Can you work these out from the model? Positions are in its coordinate system, mm. Coordinates: 2 decimals unless noted, no trailing zeros. Order: outer loops, then holes, each group sorted by start corner. A loop starts at its lowest first (then second) coordinate and runs counter-clockwise, first axis right, second up. Notation, with made-up numbers: (82.25, 34) -> (108.25, 34) arc R14 cw to (108.25, 55) -> close; hole circle Ø10 at (12, 6). An arc over 180 degrees is marked (long way). Return JSON: item names as keys, results as strings. Group by question number.
1) For pin 1 (1.6 mm diameter, centred on x = -10.5, z = 29.5, fed in from +Y); pin 2 (0.8 mm diameter, centred on y = -20.5, z = 29, fed in from -X); pin 3 (1.1 mm diameter, centred on y = -20.5, z = 29, fed in from +X); pin 4 (0.8 mm diameter, centred on x = 10.5, z = 29.5, fed in from +Y), each with a flat end and sliding along its axis, tell me the tip position at first contact or that it passes through.
2) If we section it at B-B, the plane y = 11: Please give me the cut outline in (x, z), then the cut area to 3 significant figures.
3) If we section it at A-A, the plane z = 29: Please give me the cut outline in (x, y), then the cut area to 3 significant figures.
4) If I drill on probe 1 along Y at (x, z) = (-12, 29.5), over which ranges is the centre line in solid material (lowest first)? Write a range as from..to.
from build123d import *

# Parameters (mm, degrees)
SKETCH_W        = 42
SKETCH_H        = 42
PAD_DEPTH       = 30
SKETCH001_W     = 40
SKETCH001_H     = 40
POCKET_DEPTH    = 1.5
SKETCH002_W     = 38
SKETCH002_H     = 38
POCKET001_DEPTH = 28
SKETCH003_W     = 10
SKETCH003_H     = 5
POCKET002_DEPTH = 300
SKETCH004_W     = 42
SKETCH004_H     = 42
PAD001_DEPTH    = 1.5


with BuildPart() as pocket002:
    # Sketch → Pad (new body)
    with BuildSketch(Plane.XY):
        Rectangle(SKETCH_W, SKETCH_H)
    extrude(amount=PAD_DEPTH)

    # Sketch001 → Pocket (cut)
    with BuildSketch(Plane.XY.offset(30)):
        Rectangle(SKETCH001_W, SKETCH001_H)
    extrude(amount=-POCKET_DEPTH, mode=Mode.SUBTRACT)

    # Sketch002 → Pocket001 (cut)
    with BuildSketch(Plane.XY.offset(28.5)):
        Rectangle(SKETCH002_W, SKETCH002_H)
    extrude(amount=-POCKET001_DEPTH, mode=Mode.SUBTRACT)

    # Sketch003 → Pocket002 (cut)
    with BuildSketch(Plane.XZ.offset(21)):
        with Locations((0, 27.5)):
            Rectangle(SKETCH003_W, SKETCH003_H)
    extrude(amount=-POCKET002_DEPTH, mode=Mode.SUBTRACT)


with BuildPart() as cut:
    # Pad001 base: copy of Pocket002
    add(pocket002.part)

    # Sketch004 → Pad001 (new body, symmetric)
    with BuildSketch(Plane.XY.offset(30)):
        Rectangle(SKETCH004_W, SKETCH004_H)
    extrude(amount=PAD001_DEPTH, both=True)

    # Cut: cut Pocket002
    add(pocket002.part, mode=Mode.SUBTRACT)


solid = cut.part
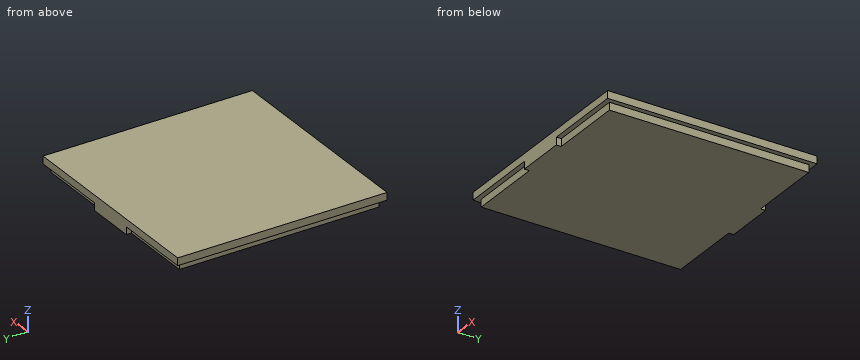
Result sheet:
{
 "1": {"pin 1": "stops at y = 21", "pin 2": "stops at x = -5", "pin 3": "stops at x = 20", "pin 4": "stops at y = 20"},
 "2": {"outline": "(-21, 30) -> (-20, 30) -> (-20, 28.5) -> (20, 28.5) -> (20, 30) -> (21, 30) -> (21, 31.5) -> (-21, 31.5) -> close", "area": "123 mm2"},
 "3": {"outline": "(-20, -20) -> (-5, -20) -> (-5, -21) -> (5, -21) -> (5, -20) -> (20, -20) -> (20, 20) -> (5, 20) -> (5, 21) -> (-5, 21) -> (-5, 20) -> (-20, 20) -> close", "area": "1,620 mm2"},
 "4": {"probe 1": "y = -20..20"}
}
